Here's the drawing with two shaded views (mm, measured from the low corner). I have some questions. A direction names the side the tool comes from. Coordinates: 2 decimals unless noted, no trailing zeros. Write each loop counter-clockwise with the first axis right and the second up, starting at its lowest first coordinate (ties: lowest second). Pieces come first, ordered by that corner, then holes. Notation, with made-up numbers: (35.25, 52.25) -> (50.25, 52.25) arc R13 ccw to (50.25, 74.25) -> close; hole circle Ø7 at (-7.5, 72.5). An arc over 180 degrees is marked (long way). Use one line per item in the form item = value.
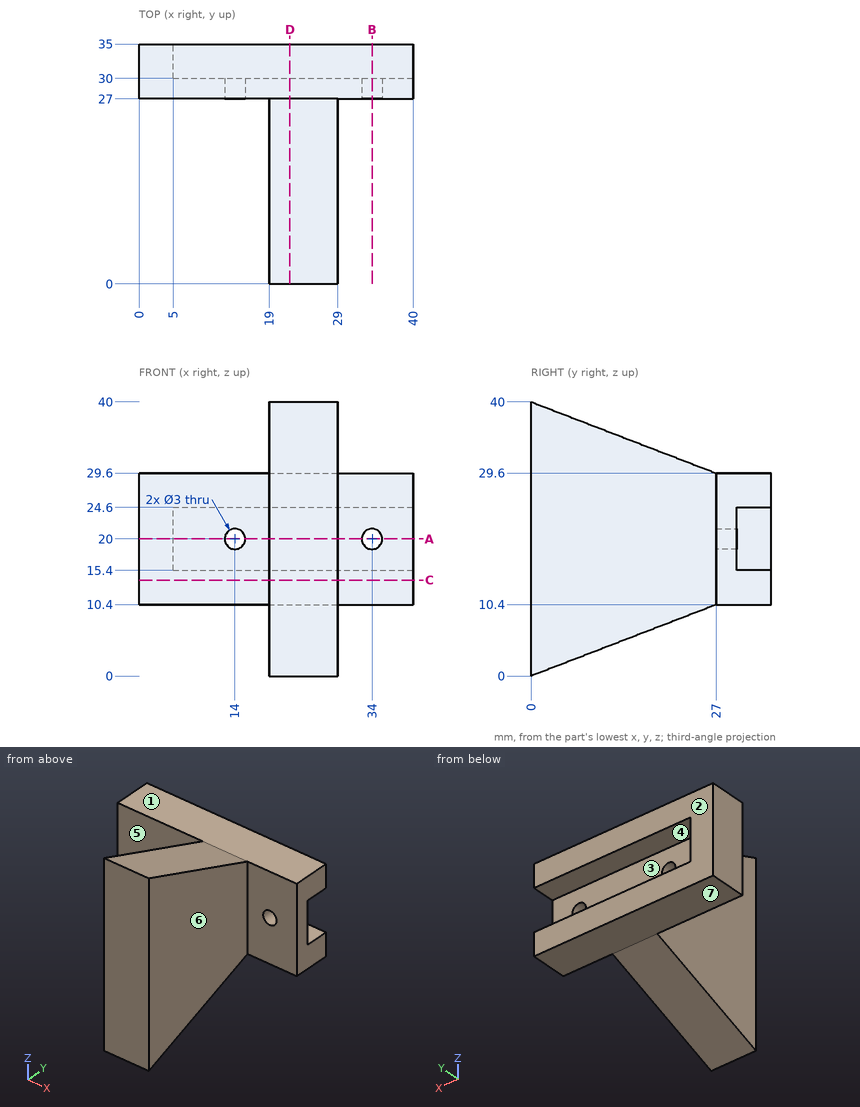
Q1. If I drill on line 1 (X direction, y = 28, z = 20); line 2 (Z direction, x = 14, y = 28); line 3 (Y direction, x = 38.5, z = 26), over which ranges is the centre line in solid material (lowest first)? Write a range as from..to.
Return value:
line_1 = 0..12.5, 15.5..32.5, 35.5..40
line_2 = 10.4..18.5, 21.5..29.6
line_3 = 27..35
Q2. Suppose I cut it at A-A (z = 20). Write out the boundary of the cut face in (x, y), then the cut area to 3 significant figures.
Return value:
outline = (0, 27) -> (12.5, 27) -> (12.5, 30) -> (5, 30) -> (5, 35) -> (0, 35) -> close; (15.5, 27) -> (19, 27) -> (19, 0) -> (29, 0) -> (29, 27) -> (32.5, 27) -> (32.5, 30) -> (15.5, 30) -> close; (35.5, 27) -> (40, 27) -> (40, 30) -> (35.5, 30) -> close
area = 397 mm2
Q3. Thinking about a two-plate mould opening in Z: for the marked faces 1, 2, 3 and 4, which applies, released by +Z, released by -Z, zero draft, split by the parting line, or undercut?
Return value:
face_1 = released by +Z
face_2 = zero draft
face_3 = undercut
face_4 = undercut
Q4. For the marked faces 5, 6 and 7, which set-ups out of +Z, -Z, +X, -X, +Y, -Y let a thin tool reach every point of the face, with its end or its side?
Return value:
face_5 = +Z, -Z, -X, -Y
face_6 = +Z, -Z, +X, -Y
face_7 = -Z, +X, -X, +Y
Q5. Suppose I cut it at B-B (x = 34). Write out the boundary of the cut face in (y, z).
Return value:
outline = (27, 10.4) -> (35, 10.4) -> (35, 15.4) -> (30, 15.4) -> (30, 18.5) -> (27, 18.5) -> close; (27, 21.5) -> (30, 21.5) -> (30, 24.6) -> (35, 24.6) -> (35, 29.6) -> (27, 29.6) -> close
Q6. Suppose I cut it at D-D (x = 22). Write out the boundary of the cut face in (y, z), then the cut area to 3 significant figures.
Return value:
outline = (0, 0) -> (27, 10.4) -> (35, 10.4) -> (35, 15.4) -> (30, 15.4) -> (30, 24.6) -> (35, 24.6) -> (35, 29.6) -> (27, 29.6) -> (0, 40) -> close
area = 907 mm2
Q7. Suppose I cut it at C-C (z = 14). Write out the boundary of the cut face in (x, y), then the cut area to 3 significant figures.
Return value:
outline = (0, 27) -> (19, 27) -> (19, 0) -> (29, 0) -> (29, 27) -> (40, 27) -> (40, 35) -> (0, 35) -> close
area = 590 mm2
Q8. Will these pins go through, and if not, where does the flat tip stop? pin 1 (1.5 mm diameter, centred on x = 19, y = 32, fed in from +Z); pin 2 (1.5 mm diameter, centred on x = 24, y = 32, fed in from -Z); pin 3 (5 mm diameter, centred on y = 12.5, z = 20.5, fed in from -X); pin 4 (2.5 mm diameter, centred on x = 14, z = 20, fed in from -Y).
Return value:
pin_1 = 29.6
pin_2 = 10.4
pin_3 = 19
pin_4 = through
